from build123d import *

# Parameters (mm, degrees)
F0_R     = 25
F1_DEPTH = 80


with BuildPart() as f1:
    # F0 (on Right) → F1 (new body)
    with BuildSketch(Plane.YZ):
        with BuildLine():
            Line((514.9215630055, -8.9879893152), (34.9946693305, -0.6108342253))
            ThreePointArc((34.9946693305, -0.6108342253), (24.6655973277, -24.8315989914), (0.3760957557, -34.9979792557))
            ThreePointArc((0.3760957557, -34.9979792557), (0.7357689155, -35.0079798205), (1.0952040016, -35.0244483385))
            Line((1.0952040016, -35.0244483385), (39.008660322, -35.6862301802))
            Line((39.008660322, -35.6862301802), (444.3213901193, -42.7609901951))
            Line((444.3213901193, -42.7609901951), (443.3615077652, -97.7526134287))
            ThreePointArc((443.3615077652, -97.7526134287), (477.7453428704, -133.3581169844), (513.3508464262, -98.9742818793))
            Line((513.3508464262, -98.9742818793), (514.9215630055, -8.9879893152))
        make_face()
        with Locations((478.3561770957, -98.363447654)):
            Circle(F0_R, mode=Mode.SUBTRACT)
        with BuildLine():
            ThreePointArc((35, 0), (34.9986673072, -0.3054287424), (34.9946693305, -0.6108342253))
            Line((34.9946693305, -0.6108342253), (514.9215630055, -8.9879893152))
            Line((514.9215630055, -8.9879893152), (515.5323972308, 26.0066800153))
            Line((515.5323972308, 26.0066800153), (0.6108342253, 34.9946693305))
            ThreePointArc((0.6108342253, 34.9946693305), (24.9637657204, 24.5318242505), (35, 0))
        make_face()
        with BuildLine():
            ThreePointArc((24.9961923789, -0.4363101609), (17.5227316075, -17.8312612289), (0, -25))
            Line((0, -25), (-24.4948974278, -25))
            ThreePointArc((-24.4948974278, -25), (-13.5110249136, -32.2870284446), (-0.6108342253, -34.9946693305))
            ThreePointArc((-0.6108342253, -34.9946693305), (-0.4934677657, -34.9965211066), (-0.3760957557, -34.9979792557))
            ThreePointArc((-0.3760957557, -34.9979792557), (0, -34.9944432379), (0.3760957557, -34.9979792557))
            ThreePointArc((0.3760957557, -34.9979792557), (24.6655973277, -24.8315989914), (34.9946693305, -0.6108342253))
            Line((34.9946693305, -0.6108342253), (24.9961923789, -0.4363101609))
        make_face()
        with BuildLine():
            ThreePointArc((0, -25), (-17.6776695297, 17.6776695297), (25, 0))
            ThreePointArc((25, 0), (24.9990480766, -0.2181633875), (24.9961923789, -0.4363101609))
            Line((24.9961923789, -0.4363101609), (34.9946693305, -0.6108342253))
            ThreePointArc((34.9946693305, -0.6108342253), (34.9986673072, -0.3054287424), (35, 0))
            ThreePointArc((35, 0), (24.9637657204, 24.5318242505), (0.6108342253, 34.9946693305))
            ThreePointArc((0.6108342253, 34.9946693305), (-24.5318242505, 24.9637657204), (-35, 0))
            ThreePointArc((-35, 0), (-32.2670219417, -13.5587350078), (-24.4948974278, -25))
            Line((-24.4948974278, -25), (0, -25))
        make_face()
        with BuildLine():
            ThreePointArc((-0.6108342253, -34.9946693305), (-13.5110249136, -32.2870284446), (-24.4948974278, -25))
            Line((-24.4948974278, -25), (-60, -25))
            Line((-60, -25), (-623.5117081128, -25))
            ThreePointArc((-623.5117081128, -25), (-613.6612070325, -35.8135916236), (-610.0951047769, -49.999819101))
            ThreePointArc((-610.0951047769, -49.999819101), (-613.6612844084, -64.1861907556), (-623.5119808251, -74.999819101))
            Line((-623.5119808251, -74.999819101), (-0.0951047769, -74.999819101))
            Line((-0.0951047769, -74.999819101), (-0.6107169229, -35.0037684849))
            Line((-0.6107169229, -35.0037684849), (-0.6108342253, -34.9946693305))
        make_face()
        with BuildLine():
            Line((-60, -25), (-24.4948974278, -25))
            ThreePointArc((-24.4948974278, -25), (-32.2670219417, -13.5587350078), (-35, 0))
            ThreePointArc((-35, 0), (-42.3223304703, -17.6776695297), (-60, -25))
        make_face()
        with BuildLine():
            ThreePointArc((-610.0951047769, -49.999819101), (-613.6612070325, -35.8135916236), (-623.5117081128, -25))
            Line((-623.5117081128, -25), (-640, -25))
            ThreePointArc((-640, -25), (-622.3838425488, -32.3558062272), (-615.0951047769, -49.999819101))
            ThreePointArc((-615.0951047769, -49.999819101), (-622.4174352472, -67.6774886306), (-640.0951047769, -74.999819101))
            Line((-640.0951047769, -74.999819101), (-623.5119808251, -74.999819101))
            ThreePointArc((-623.5119808251, -74.999819101), (-613.6612844084, -64.1861907556), (-610.0951047769, -49.999819101))
        make_face()
        with BuildLine():
            Line((-640, -25), (-623.5117081128, -25))
            ThreePointArc((-623.5117081128, -25), (-670.0951047765, -49.999655473), (-623.5119808251, -74.999819101))
            Line((-623.5119808251, -74.999819101), (-640.0951047769, -74.999819101))
            ThreePointArc((-640.0951047769, -74.999819101), (-665.0950595521, -49.9522666265), (-640, -25))
        make_face()
        with BuildLine():
            Line((1.0952040016, -35.0244483385), (-0.3974963091, -34.9983931577))
            ThreePointArc((-0.3974963091, -34.9983931577), (-0.5041137806, -35.0007966248), (-0.6107169229, -35.0037684849))
            Line((-0.6107169229, -35.0037684849), (-0.0951047769, -74.999819101))
            ThreePointArc((-0.0951047769, -74.999819101), (14.1104515348, -69.1749451733), (20.0028009778, -54.9972442157))
            ThreePointArc((20.0028009778, -54.9972442157), (14.5261693958, -41.2457915782), (1.0952040016, -35.0244483385))
        make_face()
        with BuildLine():
            Line((39.008660322, -35.6862301802), (1.0952040016, -35.0244483385))
            ThreePointArc((1.0952040016, -35.0244483385), (14.5261693958, -41.2457915782), (20.0028009778, -54.9972442157))
            ThreePointArc((20.0028009778, -54.9972442157), (25.6016517806, -41.4993509969), (39.008660322, -35.6862301802))
        make_face()
    extrude(amount=-F1_DEPTH)


solid = f1.part
Part model, mm, in its own coordinate system. A direction names the side the tool comes from. Coordinates: 2 decimals unless noted, no trailing zeros. Order: outer loops, then holes, each group sorted by start corner. A loop starts at its lowest first (then second) coordinate and runs counter-clockwise, first axis right, second up. Notation, with made-up numbers: M 26.25,-14 L 56.25,-14 A19 ccw 56.25,8 Z; hole C 59.25,32 d5. An arc over 180 degrees is marked long. Use a Markdown table: item, result.
(1) Probe L1, parallel to Y at x = -72, z = -50; L2, parallel to Y at x = -14.5, z = -49; L3, parallel to Z at x = -50, y = -451.5. List the from-to ranges inside material, lowest first.
A:
| item | result |
|---|---|
| L1 | y = -670.1 to -665.1, -615.1 to 20.7, 444.2 to 514.21 |
| L2 | y = -670.08 to -665.08, -615.12 to 21, 444.21 to 514.22 |
| L3 | z = -75 to -25 |
(2) Cut at B-B on y = -293. Write the cut outline in (x, z), then the cut area to 3 significant figures.
A:
| item | result |
|---|---|
| outline | M -80,-75 L 0,-75 L 0,-25 L -80,-25 Z |
| area | 4,000 mm^2 |
(3) Pull direction Z, two halves, no side cores. Call faces 4 (the cylindrical face through (-39.44, 453.38, -97.26)), 5 (the cylindrical face through (-39.44, 13.953, -69.33)), 6 (the flat face through (-39, -338, -25)): released by +Z, released by -Z, zero draft, split by the parting line, or undercut.
A:
| item | result |
|---|---|
| face 4 | undercut |
| face 5 | released by -Z |
| face 6 | released by +Z |
(4) Tool access for faces 1 (the flat face through (-39, -316, -75)), 2 (the flat face through (-80, -86, -29)), 3 (the cylindrical face through (-39.44, -42.129, -17.482)): list every direction of +Z, -Z, +X, -X, +Y, -Y with a clear straight run to the whole face (end or side of a thin tool).
A:
| item | result |
|---|---|
| face 1 | -Z, +X, -X |
| face 2 | +Z, -Z, -X, +Y, -Y |
| face 3 | +Z, +X, -X |
(5) Flat gauge pins, fed straight in: pin 1 (8 mm diameter, centred on x = -42, y = -425.5, fed in from +Z); pin 2 (2 mm diameter, centred on x = -14, y = -162.5, fed in from -Z); pin 3 (5 mm diameter, centred on x = -42.5, z = -34, fed in from -Y). Where does each tip first touch, or does it go through?
A:
| item | result |
|---|---|
| pin 1 | stops at z = -25 |
| pin 2 | stops at z = -75 |
| pin 3 | stops at y = -666.89 |
(6) Cut at C-C on y = 234. Write the cut outline in (x, z), then the cut area to 3 significant figures.
A:
| item | result |
|---|---|
| outline | M -80,-39.09 L 0,-39.09 L 0,30.92 L -80,30.92 Z |
| area | 5,600 mm^2 |
